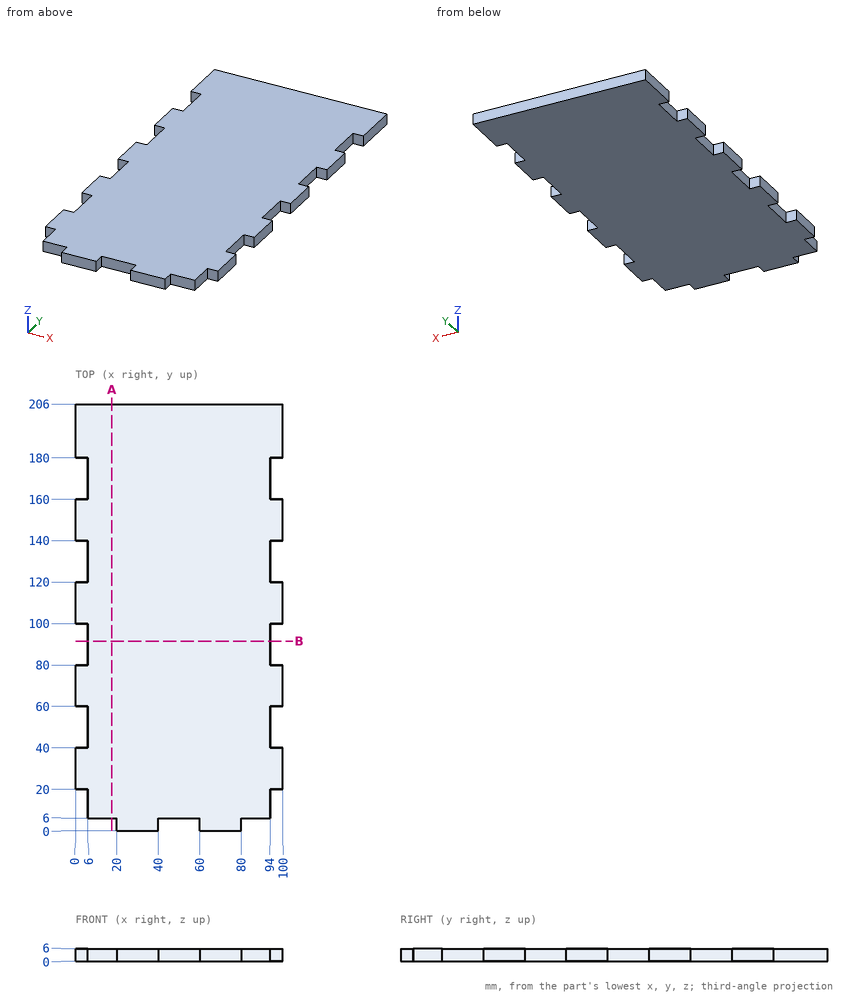
Geometry: see drawing. Coordinates: mm, zero at the bounding-box minimum. Give positions to 0.01 mm unless a question says otherwise; leave off trailing zeros. Loops run counter-clockwise (first coordinate to the right, second up) from the corner with the lowest first, then second, coordinate; pieces in that order, holes last. Notation, with made-up numbers: (-39, -7.75) - (-1, -7.75) arc R9 cw to (-1, 6.25) - close; hole circle Ø7 at (-12, 62.5). An arc over 180 degrees is marked (long way). One line per question, with ' | ' between items. Start each with the question number.
(1) Section query B-B on y = 91.5. Return loops of the section in (x, z).
(2) Contact query for flat-ended pins moving along their axis: pin 1 (1.8 mm diameter, centred on x = 4, z = 3.5, fed in from -Y); pin 2 (1 mm diameter, centred on x = 43, z = 2.5, fed in from -Y); pin 3 (3 mm diameter, centred on y = 172.5, z = 1.5, fed in from -X). Output: stop coordinate, or through.
(3) Ray query, line 1 (Y direction, x = 95.5, z = 4); line 2 (X direction, y = 87.5, z = 3.5); line 3 (Y direction, x = 9, z = 0.75). Return the intervals inside material, ascending. Write a range as from..to.
(4) Section query A-A on x = 17.5. Return loops of the section in (y, z).
The answers:
1) outline: (6, 0) - (94, 0) - (94, 6) - (6, 6) - close
2) pin 1: y = 20 | pin 2: y = 6 | pin 3: x = 6
3) line 1: 20..40, 60..80, 100..120, 140..160, 180..206 | line 2: 6..94 | line 3: 6..206
4) outline: (6, 0) - (206, 0) - (206, 6) - (6, 6) - close
